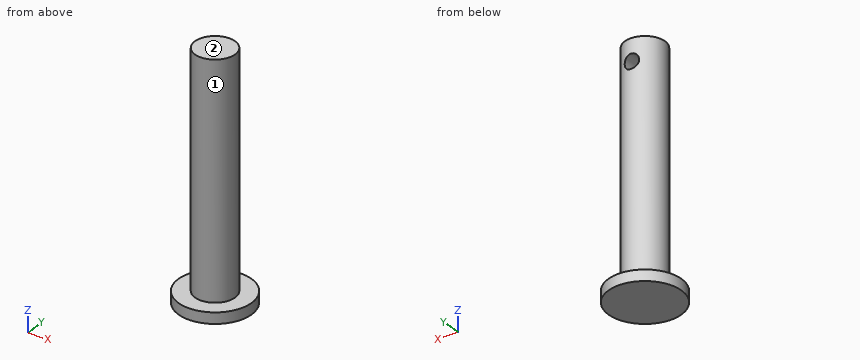
```python
from build123d import *

# Parameters (mm, degrees)
SKETCH1_R           = 5
BOSS_EXTRUDE1_DEPTH = 1.5
SKETCH2_R           = 2.75
BOSS_EXTRUDE2_DEPTH = 33
SKETCH3_R           = 1
CUT_EXTRUDE1_DEPTH  = 6


with BuildPart() as part:
    # Sketch1 → Boss-Extrude1 (new body)
    with BuildSketch(Plane.XY):
        Circle(SKETCH1_R)
    extrude(amount=BOSS_EXTRUDE1_DEPTH)

    # Sketch2 → Boss-Extrude2 (add)
    with BuildSketch(Plane.XY):
        Circle(SKETCH2_R)
    extrude(amount=BOSS_EXTRUDE2_DEPTH)

    # Sketch3 → Cut-Extrude1 (cut, through all)
    with BuildSketch(Plane(origin=(0, 0, 0), x_dir=(1, 0, 0), z_dir=(0, 1, 0))):
        with Locations((0, -30)):
            Circle(SKETCH3_R)
    extrude(amount=CUT_EXTRUDE1_DEPTH, mode=Mode.SUBTRACT)


solid = part.part
```
Design review of the part built by this model. Coordinates are the model's own, in mm. Face numbers are marked on the shaded views. A direction names the side the tool comes from. Coordinates: 2 decimals unless noted, no trailing zeros. Order: outer loops, then holes, each group sorted by start corner. A loop starts at its lowest first (then second) coordinate and runs counter-clockwise, first axis right, second up. Notation, with made-up numbers: (29.5, 44.25) - (65.5, 44.25) arc R24 ccw to (65.5, 69.25) - close; hole circle Ø4 at (14.25, 80). An arc over 180 degrees is marked (long way). Answer in a Markdown table with one row per item.
(1) Consider section B-B on y = -0.75. State the section outline as (x, z) points.
Checked values:
| item | result |
|---|---|
| outline | (-4.94, 0) - (4.94, 0) - (4.94, 1.5) - (2.65, 1.5) - (2.65, 33) - (-2.65, 33) - (-2.65, 1.5) - (-4.94, 1.5) - close |
(2) Consider section D-D on x = -2. State the section outline as (y, z) points, plus the area to 3 significant figures.
Checked values:
| item | result |
|---|---|
| outline | (-4.58, 0) - (4.58, 0) - (4.58, 1.5) - (1.89, 1.5) - (1.89, 33) - (-1.89, 33) - (-1.89, 1.5) - (-4.58, 1.5) - close |
| area | 133 mm^2 |
(3) Wall thickness on line 1 along Z through (x, y) = (0, 1.65); line 2 along X through (y, z) = (1.45, 30); line 3 along Z through (x, y) = (-4, 2.25): over which ranges is each line inside the solid? List them lowest first. Write a range as from..to.
Checked values:
| item | result |
|---|---|
| line 1 | 0..29, 31..33 |
| line 2 | -2.34..-1, 1..2.34 |
| line 3 | 0..1.5 |
(4) For the marked faces 1 and 2, list the 3-axis set-ups (+Z, -Z, +X, -X, +Y, -Y) from which the entire face can be reached by the end or side of a thin tool; tool diameter is ignored.
Checked values:
| item | result |
|---|---|
| face 1 | +Z |
| face 2 | +Z, +X, -X, +Y, -Y |
(5) Clearance check with flat-ended pins moving along their axes: pin 1 (6 mm diameter, centred on y = -3.5, z = 13, fed in from -X); pin 2 (1.6 mm diameter, centred on x = 0, z = 30, fed in from +Y); pin 3 (6 mm diameter, centred on y = -2, z = 5.5, fed in from +X). State where each tip first meets the part, or that it passes through.
Checked values:
| item | result |
|---|---|
| pin 1 | x = -2.7 |
| pin 2 | y = 0 |
| pin 3 | x = 2.75 |
(6) Consider section C-C on z = 17. State the section outline as (x, y) points.
Checked values:
| item | result |
|---|---|
| outline | circle Ø5.5 at (0, 0) |
(7) Consider section A-A on x = 0. State the section outline as (y, z) points.
Checked values:
| item | result |
|---|---|
| outline | (-5, 0) - (5, 0) - (5, 1.5) - (2.75, 1.5) - (2.75, 29) - (0, 29) - (0, 31) - (2.75, 31) - (2.75, 33) - (-2.75, 33) - (-2.75, 1.5) - (-5, 1.5) - close |
